Model file for the job. Use its own axes, mm. Face numbers are marked on the shaded views. A direction names the side the tool comes from. Give positions to 0.01 mm unless a question says otherwise; leave off trailing zeros. Write each loop counter-clockwise with the first axis right and the second up, starting at its lowest first coordinate (ties: lowest second). Pieces come first, ordered by that corner, then holes. Notation, with made-up numbers: (50, -4) - (88, -4) arc R24 ccw to (88, 26) - close; hole circle Ø4 at (86, 0.25). An arc over 180 degrees is marked (long way). One line per item, written item: value. Start each with the question number.
(1) Probe L1, parallel to X at y = 2.65, z = -10; L2, parallel to Z at x = 10, y = 1.6; L3, parallel to Z at x = -7.25, y = 0.35. List the from-to ranges inside material, lowest first.
(2) Cut at A-A, the plane z = -13.75. List the corners of the cut face in (x, y), and give its area (3 significant figures).
(3) Drop flat-ended pins along their axis: P1, Ø3, axis at x = -8.8, z = -14.12, coming from the +Y side; P2, Ø9.5, axis at x = 7, z = -3.5, coming from the +Y side; P3, Ø1.2, axis at x = 11.45, z = -14.12, coming from the -Y side. Give the stop position or say it passes through.
(4) Cut at C-C, the plane y = 2.75. List the corners of the cut face in (x, z), and give its area (3 significant figures).
(5) Cut at D-D, the plane z = -9. List the corners of the cut face in (x, y), and give its area (3 significant figures).
(6) 3-axis set-ups, long thin cutter, end or side, ignore diameter. For the marked faces 1, 2 and 3: which of +Z, -Z, +X, -X, +Y, -Y reach the whole face in a straight line?
(7) Cut at B-B, the plane z = 0. List the corners of the cut face in (x, y), and give its area (3 significant figures).
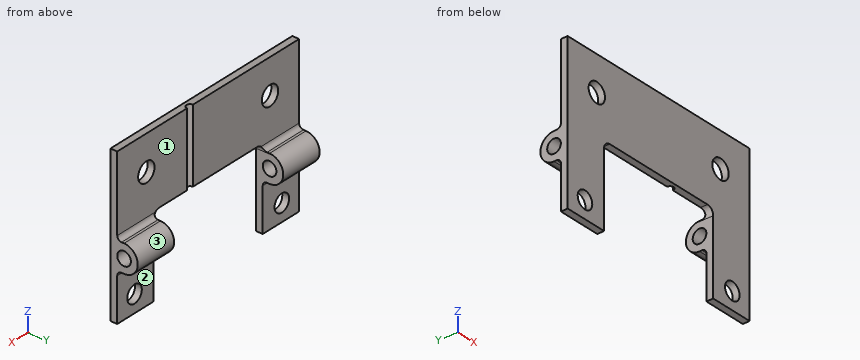
from build123d import *

# Parameters (mm, degrees)
SKETCH1_W                     = 25
SKETCH1_H                     = 10
BASE_PLATE_DEPTH              = 0.79
PINHOLDER_DEPTH               = 5
SKETCH4_R                     = 0.79
PIN_SHAFT_DEPTH               = 30.913269547
SKETCH5_R                     = 1.125
SCREW_HOLES_DEPTH             = 4
SKETCH11_R                    = 1
SET_SCREW_HOLE_DEPTH          = 1.5
MIRRORED_FILLETS_R            = 0.5
MIRRORED_FILLETS_OF_MIRROR1_R = 0.5
SPRING_GROOVE_DEPTH           = 1.5
FILLET2_R                     = 0.79
SKETCH9_R                     = 0.4


with BuildPart() as part:
    # Sketch1 → Base Plate (new body)
    with BuildSketch(Plane(origin=(0, 0, 0), x_dir=(1, 0, 0), z_dir=(0, 1, 0))):
        with Locations((1.323198198, 3.248873874)):
            Rectangle(SKETCH1_W, SKETCH1_H)
    extrude(amount=BASE_PLATE_DEPTH)

    # Sketch2 → PinHolder (add)
    with BuildSketch(Plane.ZY.offset(11.176801802)):
        with BuildLine():
            Line((-8.248873874, 0), (-8.248873874, 0.79))
            Line((-8.248873874, 0.79), (-7.458873874, 0.79))
            Line((-7.458873874, 0.79), (-7.458873874, 1.58))
            ThreePointArc((-7.458873874, 1.58), (-9.038873874, 3.16), (-10.618873874, 1.58))
            Line((-10.618873874, 1.58), (-10.618873874, 1.29))
            ThreePointArc((-10.618873874, 1.29), (-10.765320483, 0.936446609), (-11.118873874, 0.79))
            Line((-11.118873874, 0.79), (-16.118873874, 0.79))
            Line((-16.118873874, 0.79), (-16.118873874, 0))
            Line((-16.118873874, 0), (-11.426644498, 0))
            Line((-11.426644498, 0), (-8.248873874, 0))
        make_face()
    pinholder = extrude(amount=-PINHOLDER_DEPTH)

    # Sketch4 → Pin Shaft (cut, through all)
    with BuildSketch(Plane.ZY.offset(11.176801802)):
        with Locations((-9.038873874, 1.58)):
            Circle(SKETCH4_R)
    pin_shaft = extrude(amount=-PIN_SHAFT_DEPTH, mode=Mode.SUBTRACT)

    # Sketch5 → Screw Holes (cut)
    with BuildSketch(Plane(origin=(0, 0.79, 0), x_dir=(1, 0, 0), z_dir=(0, 1, 0))):
        with Locations(Location((-7.176801802, 2.248873874, 0), (0, 0, 270))):
            Circle(SKETCH5_R)
        with Locations(Location((9.823198198, 2.248873874, 0), (0, 0, 270))):
            Circle(SKETCH5_R)
    extrude(amount=-SCREW_HOLES_DEPTH, mode=Mode.SUBTRACT)

    # Sketch11 → Set Screw Hole (cut)
    with BuildSketch(Plane(origin=(0, 0.79, 0), x_dir=(1, 0, 0), z_dir=(0, 1, 0))):
        with Locations(Location((-8.801801802, 14.118873874, 0), (0, 0, 270))):
            Circle(SKETCH11_R)
    set_screw_hole = extrude(amount=-SET_SCREW_HOLE_DEPTH, mode=Mode.SUBTRACT)

    # Mirrored Fillets
    mirrored_fillets_edges = [part.edges().sort_by_distance(p)[0] for p in [
        (-8.676801802, 0.79, -7.458873874),
    ]]
    fillet(mirrored_fillets_edges, radius=MIRRORED_FILLETS_R)

    # Mirror1: PinHolder, Pin Shaft, Set Screw Hole across plane
    add(pinholder.mirror(Plane(origin=(1.323198198, 0, 0), x_dir=(0, 0, 1), z_dir=(1, 0, 0))))
    add(pin_shaft.mirror(Plane(origin=(1.323198198, 0, 0), x_dir=(0, 0, 1), z_dir=(1, 0, 0))), mode=Mode.SUBTRACT)
    add(set_screw_hole.mirror(Plane(origin=(1.323198198, 0, 0), x_dir=(0, 0, 1), z_dir=(1, 0, 0))), mode=Mode.SUBTRACT)

    # Mirrored Fillets of Mirror1
    mirrored_fillets_of_mirror1_edges = [part.edges().sort_by_distance(p)[0] for p in [
        (11.323198198, 0.79, -7.458873874),
    ]]
    fillet(mirrored_fillets_of_mirror1_edges, radius=MIRRORED_FILLETS_OF_MIRROR1_R)

    # Sketch10 → Spring Groove (cut)
    with BuildSketch(Plane(origin=(0, 0, -8.248873874), x_dir=(-1, 0, 0), z_dir=(0, 0, -1))):
        Polygon((-3.823198198, 0.79), (1.176801802, 0.79), (6.176801802, 0.79), (6.176801802, 0), (1.176801802, 0), (-3.823198198, 0), (-8.823198198, 0), (-8.823198198, 0.79), align=None)
    extrude(amount=-SPRING_GROOVE_DEPTH, mode=Mode.SUBTRACT)

    # Fillet2
    fillet2_edges = [part.edges().sort_by_distance(p)[0] for p in [
        (-6.176801802, 0.395, -6.748873874),
        (8.823198198, 0.395, -6.748873874),
    ]]
    fillet(fillet2_edges, radius=FILLET2_R)

    # Wire Groove: sweep along a path in Sketch8
    with BuildLine(Plane.XZ.offset(-0.79)) as wire_groove_path:
        Line((3.823198198, -8.248873874), (3.823198198, 1.751126126))
    # Sketch9 → Wire Groove (sweep, cut)
    with BuildSketch(Plane.XY.offset(1.751126126)):
        with Locations((3.823198198, 0.79)):
            Circle(SKETCH9_R)
    sweep(path=wire_groove_path.line, mode=Mode.SUBTRACT)


solid = part.part
Answers follow:
1. L1: x = -11.18 to -6.18, 8.82 to 13.82
1. L2: z = -10.62 to -9.83, -8.25 to -7.46
1. L3: z = -16.12 to -3.37, -1.13 to 1.75
2. outline: (-11.18, 0) - (-9.73, 0) - (-9.73, 0.79) - (-11.18, 0.79) - close; (-7.87, 0) - (-6.18, 0) - (-6.18, 0.79) - (-7.87, 0.79) - close; (8.82, 0) - (10.52, 0) - (10.52, 0.79) - (8.82, 0.79) - close; (12.38, 0) - (13.82, 0) - (13.82, 0.79) - (12.38, 0.79) - close
2. area: 4.96 mm²
3. P1: stops at y = 0.79
3. P2: stops at y = 2.66
3. P3: passes through
4. outline: (-11.18, -10.1) - (-6.18, -10.1) - (-6.18, -7.98) - (-11.18, -7.98) - close; (8.82, -10.1) - (13.82, -10.1) - (13.82, -7.98) - (8.82, -7.98) - close
4. area: 21.2 mm²
5. outline: (-11.18, 0) - (-6.18, 0) - (-6.18, 0.79) - (-11.18, 0.79) - close; (-11.18, 2.37) - (-6.18, 2.37) - (-6.18, 3.16) - (-11.18, 3.16) - close; (8.82, 0) - (13.82, 0) - (13.82, 0.79) - (8.82, 0.79) - close; (8.82, 2.37) - (13.82, 2.37) - (13.82, 3.16) - (8.82, 3.16) - close
5. area: 15.8 mm²
6. face 1: +Z, +X, -X, +Y
6. face 2: -Z, +X, -X, +Y
6. face 3: +X, -X, +Y
7. outline: (-11.18, 0) - (13.82, 0) - (13.82, 0.79) - (4.22, 0.79) arc R0.4 cw to (3.42, 0.79) - (-11.18, 0.79) - close
7. area: 19.5 mm²
